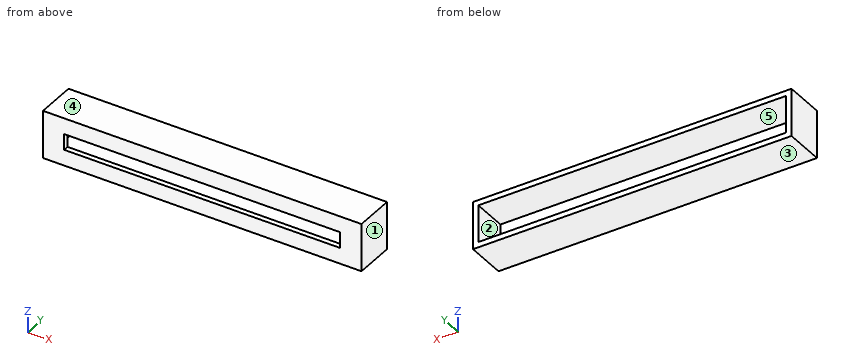
from build123d import *

# Parameters (mm, degrees)
ESQUISSE1_W             = 60
ESQUISSE1_H             = 9
BOSS_EXTRU_1_DEPTH      = 1
ESQUISSE2_W             = 60
ESQUISSE2_H             = 9
ESQUISSE2_W_2           = 58
ESQUISSE2_H_2           = 7
BOSS_EXTRU_2_DEPTH      = 6.5
ESQUISSE3_W             = 52
ESQUISSE3_H             = 3
ENL_V_MAT_EXTRU_1_DEPTH = 8.5


with BuildPart() as part:
    # Esquisse1 → Boss.-Extru.1 (new body)
    with BuildSketch(Plane(origin=(0, 0, 0), x_dir=(1, 0, 0), z_dir=(0, 1, 0))):
        with Locations((30, 4.5)):
            Rectangle(ESQUISSE1_W, ESQUISSE1_H)
    extrude(amount=BOSS_EXTRU_1_DEPTH)

    # Esquisse2 → Boss.-Extru.2 (add)
    with BuildSketch(Plane(origin=(0, 1, 0), x_dir=(1, 0, 0), z_dir=(0, 1, 0))):
        with Locations((30, 4.5)):
            Rectangle(ESQUISSE2_W, ESQUISSE2_H)
        with Locations((30, 4.5)):
            Rectangle(ESQUISSE2_W_2, ESQUISSE2_H_2, mode=Mode.SUBTRACT)
    extrude(amount=BOSS_EXTRU_2_DEPTH)

    # Esquisse3 → Enlèv. mat.-Extru.1 (cut, through all)
    with BuildSketch(Plane.XZ):
        with Locations((30, -4.5)):
            Rectangle(ESQUISSE3_W, ESQUISSE3_H)
    extrude(amount=-ENL_V_MAT_EXTRU_1_DEPTH, mode=Mode.SUBTRACT)


solid = part.part
Input: part model. Units: mm. Frame: model coordinates. Face numbers are marked on the shaded views. A direction names the side the tool comes from. Coordinates: 2 decimals unless noted, no trailing zeros. Loops run counter-clockwise (first coordinate to the right, second up) from the corner with the lowest first, then second, coordinate; pieces in that order, holes last.
(1) Section B-B on z = -5. Return the cut outline in (x, y), then the cut area to 3 significant figures.
(2) Material intervals for probe 1 along X at (y, z) = (1.75, -3.5); probe 2 along Z at (x, y) = (28, 5.5); probe 3 along Y at (x, z) = (34.5, -6.75), sorted ascending.
(3) Pull-direction query (Z, two-part tool) for the marked faces 3, 4 and 5; classes: released by +Z, released by -Z, zero draft, split by the parting line, or undercut.
(4) Section C-C on y = 0.5. Return the cut outline in (x, z).
(5) First-contact query: pin 1 Ø3 at (x, y) = (32.5, 3.5) entering from +Z; pin 2 Ø2 at (x, z) = (31.5, -5.5) entering from +Y. Flat tips, straight axial feed; report the tip coordinate or a pass-through.
(6) Section D-D on z = -1.75. Return the cut outline in (x, y).
(7) Section A-A on x = 33.5. Return the cut outline in (y, z), then the cut area to 3 significant figures.
(8) Set-up query: the marked faces 1 and 2. Return all of +Z, -Z, +X, -X, +Y, -Y with unobstructed straight access to the full face (end or side cutting, diameter ignored); none if empty.
Data:
1. outline: (0, 0) - (4, 0) - (4, 1) - (1, 1) - (1, 7.5) - (0, 7.5) - close; (56, 0) - (60, 0) - (60, 7.5) - (59, 7.5) - (59, 1) - (56, 1) - close
1. area: 21.0 mm2
2. probe 1: x = 0 to 1, 59 to 60
2. probe 2: z = -9 to -8, -1 to 0
2. probe 3: y = 0 to 1
3. face 3: released by -Z
3. face 4: released by +Z
3. face 5: undercut
4. outline: (0, -9) - (60, -9) - (60, 0) - (0, 0) - close; hole (4, -6) - (56, -6) - (56, -3) - (4, -3) - close
5. pin 1: stops at z = 0
5. pin 2: stops at y = 1
6. outline: (0, 0) - (60, 0) - (60, 7.5) - (59, 7.5) - (59, 1) - (1, 1) - (1, 7.5) - (0, 7.5) - close
7. outline: (0, -9) - (7.5, -9) - (7.5, -8) - (1, -8) - (1, -6) - (0, -6) - close; (0, -3) - (1, -3) - (1, -1) - (7.5, -1) - (7.5, 0) - (0, 0) - close
7. area: 19.0 mm2
8. face 1: +Z, -Z, +X, +Y, -Y
8. face 2: +Y
